The model under review builds one solid part; all positions refer to its coordinate system, in mm. A direction names the side the tool comes from. Give positions to 0.01 mm unless a question says otherwise; leave off trailing zeros. Loops run counter-clockwise (first coordinate to the right, second up) from the corner with the lowest first, then second, coordinate; pieces in that order, holes last. Notation, with made-up numbers: M -17,13 L 40,13 A18 cw 40,35 Z; hole C 28,78.5 d11. An arc over 180 degrees is marked long. Put each result on its own line as item: value. Start each with the question number.
```python
from build123d import *

# Parameters (mm, degrees)
F0_W     = 7.9375
F0_H     = 43.3812188
F0_W_2   = 3.175
F0_H_2   = 27.5062188
F1_DEPTH = 9.525
F2_R     = 2.15265
F3_DEPTH = 9.525
F4_R     = 3.96874


# Not quite as in the source:
# - a fillet or chamfer is up to 0.001 mm smaller than in the source, because OpenCascade refuses the exact size


with BuildPart() as f1:
    # F0 (on Top) → F1 (new body)
    with BuildSketch(Plane.XY):
        Rectangle(F0_W, F0_H)
        Rectangle(F0_W_2, F0_H_2, mode=Mode.SUBTRACT)
    extrude(amount=F1_DEPTH)

    # F2 (on face) → F3 (cut, through all)
    with BuildSketch(Plane.XY.offset(9.525)):
        with Locations((0, 17.7218594)):
            Circle(F2_R)
        with Locations((0, -17.7218594)):
            Circle(F2_R)
    extrude(amount=-F3_DEPTH, mode=Mode.SUBTRACT)

    # F4 (radius 3.96875 in the source; OpenCascade refuses exactly that, so slightly less here)
    f4_edges = [f1.edges().sort_by_distance(p)[0] for p in [
        (-3.96875, -21.690609, 4.7625),
        (3.96875, -21.690609, 4.7625),
        (3.96875, 21.690609, 4.7625),
        (-3.96875, 21.690609, 4.7625),
    ]]
    fillet(f4_edges, radius=F4_R)


solid = f1.part
```
Item 1: Clearance check with flat-ended pins moving along their axes: pin 1 Ø1.5 at (x, z) = (3, 3) entering from -Y; pin 2 Ø1 at (x, z) = (2, 3.5) entering from -Y; pin 3 Ø4 at (x, z) = (-2.5, 4.5) entering from +Y. State where each tip first meets the part, or that it passes through.
Item 2: Consider section B-B, the plane z = 2.5. Give the number of separate pieces and of enclosed holes in the cut face, plus the area to 3 significant figures.
Item 3: Consider section A-A, the plane y = 4. Write out the cut boundary in (x, z) (1 decimal), plus the area to 3 significant figures.
Item 4: Consider section C-C, the plane x = 0.75. Write out the cut boundary in (y, z) (3 decimals), plus the area to 3 significant figures.
Item 5: Draft analysis for pull direction Y (two halves, no side actions). For faces 3 (the cylindrical face through (-2.837, -20.497, 4.829)), 4 (the cylindrical face through (-2.837, 20.497, 4.829)), 5 (the flat face through (-1.588, 0, 5)), state which applies: +Y half, -Y half, draft (parallel to the pull), parting line (faces both ways), or undercut.
Item 6: Consider section D-D, the plane y = -16.5. Write out the cut boundary in (x, z) (3 decimals).
Item 7: To check wall thickness, follow L1, parallel to Y at x = 0, z = 3.25; L2, parallel to X at y = 6, z = 5; L3, parallel to Y at x = 1.5, z = 1.75. State the ranges of each line that lie inside material, in increasing order. Write a range as [from, to].
Item 8: Tool access review of faces 1 (the flat face through (2, 0, 9.525)), 2 (the flat face through (0, -13.753, 5)): name each direction out of +Z, -Z, +X, -X, +Y, -Y from which nothing blocks a thin tool from reaching the whole face with its end or side.
Report:
1. pin 1: y = -20.99
1. pin 2: y = -21.4
1. pin 3: y = 21.66
2. separate pieces: 1
2. enclosed holes: 3
2. area: 214 mm²
3. outline: M -4,0 L -1.6,0 L -1.6,9.5 L -4,9.5 Z; M 1.6,0 L 4,0 L 4,9.5 L 1.6,9.5 Z
3. area: 45.4 mm²
4. outline: M -21.619,0 L -19.74,0 L -19.74,9.525 L -21.619,9.525 Z; M -15.704,0 L -13.753,0 L -13.753,9.525 L -15.704,9.525 Z; M 13.753,0 L 15.704,0 L 15.704,9.525 L 13.753,9.525 Z; M 19.74,0 L 21.619,0 L 21.619,9.525 L 19.74,9.525 Z
4. area: 73.0 mm²
5. face 3: -Y half
5. face 4: +Y half
5. face 5: undercut
6. outline: M -3.969,0 L -1.772,0 L -1.772,9.525 L -3.969,9.525 Z; M 1.772,0 L 3.969,0 L 3.969,9.525 L 1.772,9.525 Z
7. L1: [-21.69, -19.87], [-15.57, -13.75], [13.75, 15.57], [19.87, 21.69]
7. L2: [-3.97, -1.59], [1.59, 3.97]
7. L3: [-21.4, -19.27], [-16.18, -13.75], [13.75, 16.18], [19.27, 21.4]
8. face 1: +Z, +X, -X, +Y, -Y
8. face 2: +Z, -Z
